```python
from build123d import *

# Parameters (mm, degrees)
F1_DEPTH        = 215
F0_W            = 7
F0_H            = 48
F2_DEPTH        = 202
F4_D            = 8
F4_CBORE_D      = 46
F4_CBORE_DEPTH  = 6
F5_D            = 10
F5_CBORE_D      = 46
F5_CBORE_DEPTH  = 5.5
F9_D            = 2.6
F9_DEPTH        = 8
F9_TIP          = 0.7811188047
F9_ON_F6_D      = 2.6
F9_ON_F6_DEPTH  = 8
F9_ON_F6_TIP    = 0.7811188047
F9_ON_F7_D      = 2.6
F9_ON_F7_DEPTH  = 8
F9_ON_F7_TIP    = 0.7811188047
F10_R           = 3
F11_SIZE        = 2
F14_D           = 2.6
F14_DEPTH       = 8
F14_TIP         = 0.7811188047
F15_D           = 8
F15_DEPTH       = 14
F15_CBORE_D     = 30
F15_CBORE_DEPTH = 5
F15_TIP         = 2.4034424761
F17_D           = 2
F19_D           = 5
F19_DEPTH       = 10
F19_TIP         = 1.5021515476


# Not quite as in the source:
# - a feature names something its author has since deleted; it is built from what else it names


with BuildPart() as f1:
    # F0 (on Right) → F1 (new body, symmetric)
    with BuildSketch(Plane.YZ):
        Polygon((0, 24), (0, 30), (-6.5, 30), (-6.5, 17.6169319153), (-6.5, -16.0151308179), (-6.5, -17.6169319153), (-6.5, -30), (0, -30), (0, -24), align=None)
    extrude(amount=F1_DEPTH, both=True)

    # F0 (on Right) → F2 (join, symmetric)
    with BuildSketch(Plane.YZ):
        Polygon((0, 24), (0, 30), (-6.5, 30), (-6.5, 17.6169319153), (-6.5, -16.0151308179), (-6.5, -17.6169319153), (-6.5, -30), (0, -30), (0, -24), align=None)
        with Locations((3.5, 0)):
            Rectangle(F0_W, F0_H)
    extrude(amount=F2_DEPTH, both=True)

    # F4 (through all)
    with Locations(Plane.XZ.offset(6.5)):
        with Locations((0, 0)):
            CounterBoreHole(F4_D / 2, F4_CBORE_D / 2, F4_CBORE_DEPTH)

    # F5 (through all)
    with Locations(Plane.XZ.offset(6.5)):
        with Locations((140, 0), (-140, 0)):
            CounterBoreHole(F5_D / 2, F5_CBORE_D / 2, F5_CBORE_DEPTH)

    # F9
    with Locations(Plane(origin=(-202, 0, 0), x_dir=(0, -1, 0), z_dir=(-1, 0, 0))):
        with Locations((-4, 14), (-4, -14)):
            Hole(F9_D / 2, depth=F9_DEPTH)
            with Locations((0, 0, -(F9_DEPTH + F9_TIP / 2))):  # 118° drill point
                Cone(0, F9_D / 2, F9_TIP, mode=Mode.SUBTRACT)

    # F9 on F6
    with Locations(Plane(origin=(0, 0, -24), x_dir=(1, 0, 0), z_dir=(0, 0, -1))):
        with Locations((-170, -4), (0, -4), (170, -4)):
            Hole(F9_ON_F6_D / 2, depth=F9_ON_F6_DEPTH)
            with Locations((0, 0, -(F9_ON_F6_DEPTH + F9_ON_F6_TIP / 2))):  # 118° drill point
                Cone(0, F9_ON_F6_D / 2, F9_ON_F6_TIP, mode=Mode.SUBTRACT)

    # F9 on F7
    with Locations(Plane.YZ.offset(202)):
        with Locations((4.5, -14), (4.5, 14)):
            Hole(F9_ON_F7_D / 2, depth=F9_ON_F7_DEPTH)
            with Locations((0, 0, -(F9_ON_F7_DEPTH + F9_ON_F7_TIP / 2))):  # 118° drill point
                Cone(0, F9_ON_F7_D / 2, F9_ON_F7_TIP, mode=Mode.SUBTRACT)

    # F10
    f10_edges = [f1.edges().sort_by_distance(p)[0] for p in [
        (215, -3.25, -30),
        (-215, -3.25, -30),
        (215, -3.25, 30),
        (-215, -3.25, 30),
    ]]
    fillet(f10_edges, radius=F10_R)

    # F11
    f11_edges = [f1.edges().sort_by_distance(p)[0] for p in [
        (-215, -6.5, 0),
        (0, -6.5, -30),
        (215, -6.5, 0),
        (0, -6.5, 30),
    ]]
    chamfer(f11_edges, length=F11_SIZE)

    # F14
    with Locations(Plane.XY.offset(24)):
        with Locations((0, 4), (-170, 4), (170, 4)):
            Hole(F14_D / 2, depth=F14_DEPTH)
            with Locations((0, 0, -(F14_DEPTH + F14_TIP / 2))):  # 118° drill point
                Cone(0, F14_D / 2, F14_TIP, mode=Mode.SUBTRACT)

    # F15
    with Locations(Plane(origin=(0, 7, 0), x_dir=(-1, 0, 0), z_dir=(0, 1, 0))):
        with Locations((-140, 0), (0, 0), (140, 0)):
            CounterBoreHole(F15_D / 2, F15_CBORE_D / 2, F15_CBORE_DEPTH, depth=F15_DEPTH)
            with Locations((0, 0, -(F15_DEPTH + F15_TIP / 2))):  # 118° drill point
                Cone(0, F15_D / 2, F15_TIP, mode=Mode.SUBTRACT)

    # F17 (through all)
    with Locations(Plane(origin=(0, 7, 0), x_dir=(-1, 0, 0), z_dir=(0, 1, 0))):
        with Locations((177, 0)):
            Hole(F17_D / 2)

    # F19
    with Locations(Plane(origin=(0, 7, 0), x_dir=(-1, 0, 0), z_dir=(0, 1, 0))):
        with Locations((177, 0)):
            Hole(F19_D / 2, depth=F19_DEPTH)
            with Locations((0, 0, -(F19_DEPTH + F19_TIP / 2))):  # 118° drill point
                Cone(0, F19_D / 2, F19_TIP, mode=Mode.SUBTRACT)


solid = f1.part
```
Geometry check sheet. Reference: the model listing, model coordinates, mm. A direction names the side the tool comes from. Round coordinates to 2 decimals unless told otherwise and drop trailing zeros. Loops run counter-clockwise (first coordinate to the right, second up) from the corner with the lowest first, then second, coordinate; pieces in that order, holes last. Notation, with made-up numbers: M 80,66 L 86,66 A22 cw 86,91 Z; hole C 78,41.5 d1. An arc over 180 degrees is marked long. Return JSON: item names as keys, results as strings. Group by question number.
(1) Section check A-A, the plane x = -140. Enter the section's corners in (y, z), and give its area (3 significant figures).
(2) Scan lines: line 1 along Z through (x, y) = (139, -2); line 2 along Z through (x, y) = (140, 0.9); line 3 along Y through (x, z) = (-170, 18). Record each from-to range of solid material in increasing order. Write a range as [from, to].
(3) Go/stop test with flat-tipped pins: pin 1 (2.5 mm diameter, centred on y = 4, z = -14, fed in from -X); pin 2 (2.5 mm diameter, centred on x = 0, y = 4, fed in from +Z); pin 3 (6 mm diameter, centred on x = 30.5, y = 4.5, fed in from +Z). Record where each tip stops, or that it passes through.
(4) Mould release check, pull along Z, two halves, no side actions. Record for faces 5 (the face through (-2.994, -3.542, 22.804)), 6 (the face through (3, 3, 24)), 7 (the face through (202, 3, 0)): pulls with the +Z half, pulls with the -Z half, needs draft (parallel to the pull), parting line crosses it, or undercut.
(5) Section check B-B, the plane x = 37.5. Enter the section's corners in (y, z).
(6) Set-up check for faces 1 (the face through (-202, 3, 0)), 2 (the face through (-140.3, -1, 5.4)), 3 (the face through (154.985, 4.535, 0.66)), 4 (the face through (3, 3, -24)): record each of +Z, -Z, +X, -X, +Y, -Y from which the full face is reachable in a straight line by a thin tool's end or side.
Data:
{
 "1": {"outline": "M -6.5,-28 L -4.5,-30 L 0,-30 L 0,-24 L 7,-24 L 7,-15 L 2,-15 L 2,-5 L -1,-5 L -1,-23 L -6.5,-23 Z; M -6.5,23 L -1,23 L -1,5 L 2,5 L 2,15 L 7,15 L 7,24 L 0,24 L 0,30 L -4.5,30 L -6.5,28 Z", "area": "289 mm²"},
 "2": {"line 1": "[-30, -22.98], [22.98, 30]", "line 2": "[-24, -5], [5, 24]", "line 3": "[-6.5, 2.7], [5.3, 7]"},
 "3": {"pin 1": "x = -193.97", "pin 2": "z = 15.97", "pin 3": "z = 24"},
 "4": {"face 5": "undercut", "face 6": "pulls with the +Z half", "face 7": "needs draft"},
 "5": {"outline": "M -6.5,-28 L -4.5,-30 L 0,-30 L 0,-24 L 7,-24 L 7,24 L 0,24 L 0,30 L -4.5,30 L -6.5,28 Z"},
 "6": {"face 1": "+Z, -Z, -X, +Y", "face 2": "-Y", "face 3": "+Y", "face 4": "-Z, +X, -X, +Y"}
}
